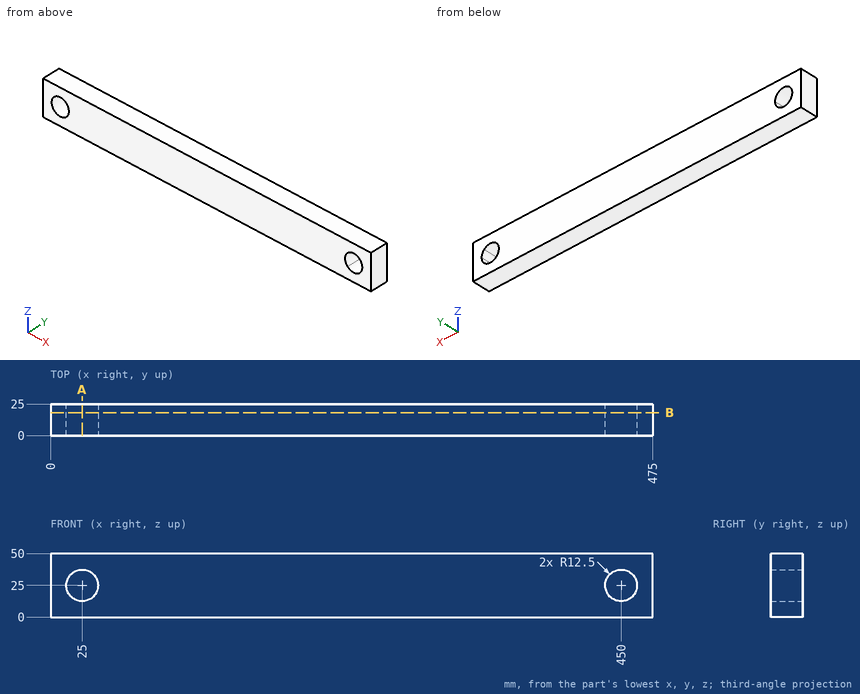
Study the drawing (mm; zero at the part's minimum x, y, z) and answer. Coordinates: 2 decimals unless noted, no trailing zeros. Write each loop counter-clockwise with the first axis right and the second up, starting at its lowest first coordinate (ties: lowest second). Pieces come first, ordered by that corner, then holes. Notation, with made-up numbers: (-11, 51) - (15, 51) arc R14 ccw to (15, 64) - close; hole circle Ø3 at (11, 78.5). An arc over 180 degrees is marked (long way). Put each result on its own line as item: value.
1. A flat-ended cylindrical pin translates along its axis: pin 1 Ø8 at (y, z) = (21.5, 24) entering from -X. Find the tip coordinate at first contact, or state that the pin passes through.
Answer sheet:
pin 1: stops at x = 0
2. The part is cut by section B-B on y = 18.25. Give the vertices of the cut face in (x, z), plus the area to 3 significant figures.
Answer sheet:
outline: (0, 0) - (475, 0) - (475, 50) - (0, 50) - close; hole (33.84, 16.16) arc R12.5 ccw to (37.5, 25) arc R12.5 ccw (long way) to start; hole (458.84, 33.84) arc R12.5 ccw (long way) to (462.5, 25) arc R12.5 ccw to start
area: 22,800 mm^2
3. The part is cut by section A-A on x = 25. Give the vertices of the cut face in (y, z), plus the area to 3 significant figures.
Answer sheet:
outline: (0, 0) - (25, 0) - (25, 12.5) - (0, 12.5) - close; (0, 37.5) - (25, 37.5) - (25, 50) - (0, 50) - close
area: 625 mm^2
4. Find the intervals of material crossed by line 1 along X through (y, z) = (22, 23); line 2 along X through (y, z) = (5, 22.5); line 3 along Z through (x, y) = (22, 2.5), in increasing order. Write a range as from..to.
Answer sheet:
line 1: x = 0..12.66, 37.34..437.66, 462.34..475
line 2: x = 0..12.75, 37.25..437.75, 462.25..475
line 3: z = 0..12.87, 37.13..50
